Input: part model. Units: mm. Frame: model coordinates. A direction names the side the tool comes from. Give positions to 0.01 mm unless a question says otherwise; leave off trailing zeros. Order: outer loops, then holes, each group sorted by start corner. A loop starts at its lowest first (then second) coordinate and runs counter-clockwise, first axis right, second up. Notation, with made-up numbers: M 38.25,8 L 55.25,8 A18 cw 55.25,35 Z; hole C 40,82 d10. An arc over 180 degrees is marked long. Use a Markdown table: item, result.
from build123d import *

# Parameters (mm, degrees)
SKETCH_1_W          = 400
SKETCH_1_H          = 110
EXTRUDE_1_DEPTH     = 8
SKETCH_2_W          = 15
SKETCH_2_H          = 2.5
CUT_EXTRUDE_1_DEPTH = 7
CUT_EXTRUDE_2_DEPTH = 9
SKETCH_8_R          = 1.5
CUT_EXTRUDE_4_DEPTH = 111
SKETCH_11_R         = 1.5
CUT_EXTRUDE_6_DEPTH = 10
SKETCH_12_R         = 1.5
CUT_EXTRUDE_7_DEPTH = 10
SKETCH_13_R         = 1.5
CUT_EXTRUDE_8_DEPTH = 10
SKETCH_14_R         = 1.5
CUT_EXTRUDE_9_DEPTH = 9


with BuildPart() as part:
    # 草图1 → 凸台-拉伸1 (new body)
    with BuildSketch(Plane(origin=(0, 0, 0), x_dir=(1, 0, 0), z_dir=(0, 1, 0))):
        Rectangle(SKETCH_1_W, SKETCH_1_H)
    extrude(amount=EXTRUDE_1_DEPTH)

    # 草图2 → 切除-拉伸1 (cut)
    with BuildSketch(Plane(origin=(0, 8, 0), x_dir=(1, 0, 0), z_dir=(0, 1, 0))):
        with Locations((-172.5, 51.25)):
            Rectangle(SKETCH_2_W, SKETCH_2_H)
        with Locations((-157.5, 51.25)):
            Rectangle(SKETCH_2_W, SKETCH_2_H)
        with Locations((-157.5, 48.75)):
            Rectangle(SKETCH_2_W, SKETCH_2_H)
        with Locations((-172.5, 48.75)):
            Rectangle(SKETCH_2_W, SKETCH_2_H)
        with Locations((-172.5, -48.75)):
            Rectangle(SKETCH_2_W, SKETCH_2_H)
        with Locations((-172.5, -51.25)):
            Rectangle(SKETCH_2_W, SKETCH_2_H)
        with Locations((-157.5, -51.25)):
            Rectangle(SKETCH_2_W, SKETCH_2_H)
        with Locations((-157.5, -48.75)):
            Rectangle(SKETCH_2_W, SKETCH_2_H)
        with Locations((172.5, 51.25)):
            Rectangle(SKETCH_2_W, SKETCH_2_H)
        with Locations((157.5, 51.25)):
            Rectangle(SKETCH_2_W, SKETCH_2_H)
        with Locations((157.5, 48.75)):
            Rectangle(SKETCH_2_W, SKETCH_2_H)
        with Locations((172.5, 48.75)):
            Rectangle(SKETCH_2_W, SKETCH_2_H)
        with Locations((157.5, -48.75)):
            Rectangle(SKETCH_2_W, SKETCH_2_H)
        with Locations((157.5, -51.25)):
            Rectangle(SKETCH_2_W, SKETCH_2_H)
        with Locations((172.5, -51.25)):
            Rectangle(SKETCH_2_W, SKETCH_2_H)
        with Locations((172.5, -48.75)):
            Rectangle(SKETCH_2_W, SKETCH_2_H)
    extrude(amount=-CUT_EXTRUDE_1_DEPTH, mode=Mode.SUBTRACT)

    # 草图3 → 切除-拉伸2 (cut, through all)
    with BuildSketch(Plane(origin=(0, 8, 0), x_dir=(1, 0, 0), z_dir=(0, 1, 0))):
        with BuildLine():
            Line((-82, 40), (-82, 0))
            Line((-82, 0), (-75, 0))
            Line((-75, 0), (-75, 47))
            ThreePointArc((-75, 47), (-79.949747468, 44.949747468), (-82, 40))
        make_face()
        with BuildLine():
            Line((-75, 47), (-75, 0))
            Line((-75, 0), (-68, 0))
            Line((-68, 0), (-68, 40))
            ThreePointArc((-68, 40), (-70.050252532, 44.949747468), (-75, 47))
        make_face()
        with BuildLine():
            Line((-75, 0), (-82, 0))
            Line((-82, 0), (-82, -40))
            ThreePointArc((-82, -40), (-79.949747468, -44.949747468), (-75, -47))
            Line((-75, -47), (-75, 0))
        make_face()
        with BuildLine():
            Line((-68, 0), (-75, 0))
            Line((-75, 0), (-75, -47))
            ThreePointArc((-75, -47), (-70.050252532, -44.949747468), (-68, -40))
            Line((-68, -40), (-68, 0))
        make_face()
        with BuildLine():
            Line((-7, 40), (-7, 0))
            Line((-7, 0), (0, 0))
            Line((0, 0), (0, 47))
            ThreePointArc((0, 47), (-4.949747468, 44.949747468), (-7, 40))
        make_face()
        with BuildLine():
            Line((0, 47), (0, 0))
            Line((0, 0), (7, 0))
            Line((7, 0), (7, 40))
            ThreePointArc((7, 40), (4.949747468, 44.949747468), (0, 47))
        make_face()
        with BuildLine():
            Line((0, 0), (-7, 0))
            Line((-7, 0), (-7, -40))
            ThreePointArc((-7, -40), (-4.949747468, -44.949747468), (0, -47))
            Line((0, -47), (0, 0))
        make_face()
        with BuildLine():
            Line((7, 0), (0, 0))
            Line((0, 0), (0, -47))
            ThreePointArc((0, -47), (4.949747468, -44.949747468), (7, -40))
            Line((7, -40), (7, 0))
        make_face()
        with BuildLine():
            Line((68, 40), (68, 0))
            Line((68, 0), (75, 0))
            Line((75, 0), (75, 47))
            ThreePointArc((75, 47), (70.050252532, 44.949747468), (68, 40))
        make_face()
        with BuildLine():
            Line((75, 47), (75, 0))
            Line((75, 0), (82, 0))
            Line((82, 0), (82, 40))
            ThreePointArc((82, 40), (79.949747468, 44.949747468), (75, 47))
        make_face()
        with BuildLine():
            Line((75, 0), (68, 0))
            Line((68, 0), (68, -40))
            ThreePointArc((68, -40), (70.050252532, -44.949747468), (75, -47))
            Line((75, -47), (75, 0))
        make_face()
        with BuildLine():
            Line((82, 0), (75, 0))
            Line((75, 0), (75, -47))
            ThreePointArc((75, -47), (79.949747468, -44.949747468), (82, -40))
            Line((82, -40), (82, 0))
        make_face()
    extrude(amount=-CUT_EXTRUDE_2_DEPTH, mode=Mode.SUBTRACT)

    # 草图8 → 切除-拉伸4 (cut, through all)
    with BuildSketch(Plane.XY.offset(55)):
        with Locations((165, 4.5)):
            Circle(SKETCH_8_R)
        with Locations((-165, 4.5)):
            Circle(SKETCH_8_R)
    extrude(amount=-CUT_EXTRUDE_4_DEPTH, mode=Mode.SUBTRACT)

    # 草图11 → 切除-拉伸6 (cut)
    with BuildSketch(Plane(origin=(0, 8, 0), x_dir=(1, 0, 0), z_dir=(0, 1, 0))):
        with Locations((126, 24.5)):
            Circle(SKETCH_11_R)
        with Locations((185, 24.5)):
            Circle(SKETCH_11_R)
        with Locations((185, -24.5)):
            Circle(SKETCH_11_R)
        with Locations((126, -24.5)):
            Circle(SKETCH_11_R)
    extrude(amount=-CUT_EXTRUDE_6_DEPTH, mode=Mode.SUBTRACT)

    # 草图12 → 切除-拉伸7 (cut)
    with BuildSketch(Plane(origin=(0, 8, 0), x_dir=(1, 0, 0), z_dir=(0, 1, 0))):
        with Locations((61, 19.5)):
            Circle(SKETCH_12_R)
        with Locations((95, 19.5)):
            Circle(SKETCH_12_R)
        with Locations((95, -19.5)):
            Circle(SKETCH_12_R)
        with Locations((61, -19.5)):
            Circle(SKETCH_12_R)
    extrude(amount=-CUT_EXTRUDE_7_DEPTH, mode=Mode.SUBTRACT)

    # 草图13 → 切除-拉伸8 (cut)
    with BuildSketch(Plane(origin=(0, 8, 0), x_dir=(1, 0, 0), z_dir=(0, 1, 0))):
        with Locations((-34, 46.75)):
            Circle(SKETCH_13_R)
        with Locations((40, 46.75)):
            Circle(SKETCH_13_R)
        with Locations((40, -46.75)):
            Circle(SKETCH_13_R)
        with Locations((-34, -46.75)):
            Circle(SKETCH_13_R)
    extrude(amount=-CUT_EXTRUDE_8_DEPTH, mode=Mode.SUBTRACT)

    # 草图14 → 切除-拉伸9 (cut, through all)
    with BuildSketch(Plane(origin=(0, 8, 0), x_dir=(1, 0, 0), z_dir=(0, 1, 0))):
        with Locations((-91, -24.5)):
            Circle(SKETCH_14_R)
        with Locations((-91, -34.5)):
            Circle(SKETCH_14_R)
        with Locations((-59, -34.5)):
            Circle(SKETCH_14_R)
        with Locations((-59, -24.5)):
            Circle(SKETCH_14_R)
    extrude(amount=-CUT_EXTRUDE_9_DEPTH, mode=Mode.SUBTRACT)


solid = part.part
1) Reachability of faces 1 (the face through (-7, 4, -1)), 2 (the face through (-165, 7, -47.5)), 3 (the face through (-3, 4, 55)) from +Z, -Z, +X, -X, +Y, -Y: full face, straight path, thin tool, end or side. Return the list, or none.
Response values:
| item | result |
|---|---|
| face 1 | +Y, -Y |
| face 2 | +Y |
| face 3 | +Z, +X, -X, +Y, -Y |
2) Cut plane A-A on z = -35. Return loops of the section in (x, y), and give its area (3 significant figures).
Response values:
| item | result |
|---|---|
| outline | M -200,0 L -82,0 L -82,8 L -200,8 Z; M -68,0 L -7,0 L -7,8 L -68,8 Z; M 7,0 L 68,0 L 68,8 L 7,8 Z; M 82,0 L 200,0 L 200,8 L 82,8 Z; hole C -165,4.5 d3; hole C 165,4.5 d3 |
| area | 2,850 mm² |
3) Mould query, pull axis X, two halves, no side actions, for faces 4 (the face through (-68, 4, 1)), 5 (the face through (-200, 4, 1)), 6 (the face through (200, 4, 1)), 7 (the face through (42, 0, -1)). Classes: released by +X, released by -X, zero draft, split by the parting line, or undercut.
Response values:
| item | result |
|---|---|
| face 4 | undercut |
| face 5 | released by -X |
| face 6 | released by +X |
| face 7 | zero draft |
4) Material intervals for line 1 (Z direction, x = -59, y = 2); line 2 (X direction, y = 2.5, z = -33.5); line 3 (Z direction, x = 61, y = 5), sorted ascending. Write a range as from..to.
Response values:
| item | result |
|---|---|
| line 1 | z = -55..23, 26..33, 36..55 |
| line 2 | x = -200..-82, -68..-7, 7..68, 82..200 |
| line 3 | z = -55..-21, -18..18, 21..55 |
5) First-contact query: pin 1 Ø2.5 at (x, z) = (-34, 46.75) entering from +Y. Flat tip, straight axial feed; report the tip coordinate or a pass-through.
Response values:
| item | result |
|---|---|
| pin 1 | passes through |
